Source: CAD feature listing. Evaluate the final solid. Frame: model axes, mm. Coordinates: 2 decimals unless noted, no trailing zeros. Loops run counter-clockwise (first coordinate to the right, second up) from the corner with the lowest first, then second, coordinate; pieces in that order, holes last. Notation, with made-up numbers: (25.25, 60.5) - (59.25, 60.5) arc R36 ccw to (59.25, 98.5) - close; hole circle Ø3 at (-34, 33.5). An arc over 180 degrees is marked (long way). Use one line per item in the form item = value. Start each with the question number.
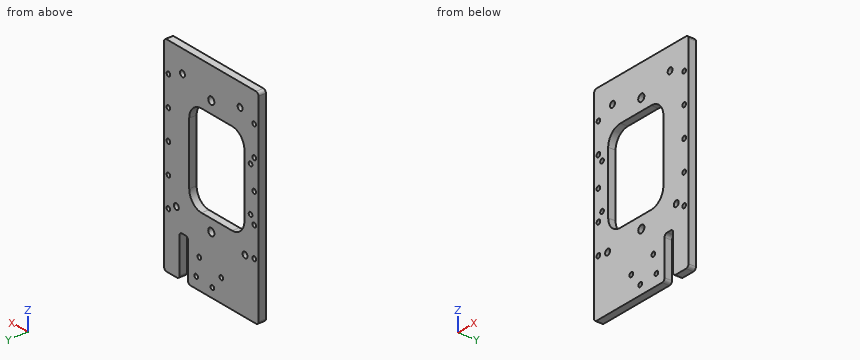
from build123d import *

# Parameters (mm, degrees)
SKETCH_1_W          = 77
SKETCH_1_H          = 138
SKETCH_1_R          = 2.5
SKETCH_1_W_2        = 45
SKETCH_1_H_2        = 62
EXTRUDE_1_DEPTH     = 5
SKETCH_7_W          = 7
SKETCH_7_H          = 28
CUT_EXTRUDE_1_DEPTH = 6
MM_CLEARANCE_0_D    = 4
FILLET_1_R          = 10
FILLET_2_R          = 2
MM_TRANSITIONAL_0_D = 3
MM_CLEARANCE_0_2_D  = 3


with BuildPart() as part:
    # 草图1 → 凸台-拉伸1 (new body)
    with BuildSketch(Plane(origin=(0, 0, 0), x_dir=(1, 0, 0), z_dir=(0, 1, 0))):
        with Locations((0, 9)):
            Rectangle(SKETCH_1_W, SKETCH_1_H)
        with Locations((0, 39)):
            Circle(SKETCH_1_R, mode=Mode.SUBTRACT)
        with Locations((0, -39)):
            Circle(SKETCH_1_R, mode=Mode.SUBTRACT)
        with Locations((-4.5, 0)):
            Rectangle(SKETCH_1_W_2, SKETCH_1_H_2, mode=Mode.SUBTRACT)
    extrude(amount=EXTRUDE_1_DEPTH)

    # 草图7 → 切除-拉伸1 (cut, through all)
    with BuildSketch(Plane(origin=(0, 5, 0), x_dir=(1, 0, 0), z_dir=(0, 1, 0))):
        with Locations((22.5, 64)):
            Rectangle(SKETCH_7_W, SKETCH_7_H)
    extrude(amount=-CUT_EXTRUDE_1_DEPTH, mode=Mode.SUBTRACT)

    # mm Clearance _0 (through all)
    with Locations(Plane(origin=(0, 0, 0), x_dir=(-1, 0, 0), z_dir=(0, -1, 0))):
        with Locations((-28.5, 36), (27.5, 41), (23.5, -45), (-23.5, -45)):
            Hole(MM_CLEARANCE_0_D / 2)

    # 圆角1
    fillet_1_edges = [part.edges().sort_by_distance(p)[0] for p in [
        (-27, 2.5, -31),
        (-27, 2.5, 31),
        (18, 2.5, 31),
        (18, 2.5, -31),
    ]]
    fillet(fillet_1_edges, radius=FILLET_1_R)

    # 圆角2
    fillet_2_edges = [part.edges().sort_by_distance(p)[0] for p in [
        (19, 2.5, -50),
        (19, 2.5, -78),
        (26, 2.5, -78),
        (26, 2.5, -50),
        (38.5, 2.5, 60),
        (-38.5, 2.5, 60),
        (-38.5, 2.5, -78),
        (38.5, 2.5, -78),
    ]]
    fillet(fillet_2_edges, radius=FILLET_2_R)

    # 大小mm Transitional 暗销孔0 (through all)
    with Locations(Plane(origin=(0, 5, 0), x_dir=(1, 0, 0), z_dir=(0, 1, 0))):
        with Locations((-31.999999999, 15), (-31.999999999, -15), (-8.142857142, 62.612808878), (-0.857142857, 71.612808878), (12.309431, 70.612808878), (9.80943136, 58.112808878)):
            Hole(MM_TRANSITIONAL_0_D / 2)

    # mm Clearance _0 2 (through all)
    with Locations(Plane(origin=(0, 5, 0), x_dir=(1, 0, 0), z_dir=(0, 1, 0))):
        with Locations((-35, 0), (-35, 20), (-35, 40), (-35, -40), (-35, -20), (35, 40), (35, 20), (35, 0), (35, -20), (35, -40)):
            Hole(MM_CLEARANCE_0_2_D / 2)


solid = part.part
(1) Contact query for a flat-ended pin moving along its axis: pin 1 (0.9 mm diameter, centred on x = 22, y = 1.5, fed in from -Z). Output: stop coordinate, or through.
(2) Cut plane C-C, the plane y = 2.7. State how many separate pieces and enclosed holes the cut face has, plus the area to 3 significant figures.
(3) Cut plane B-B, the plane x = -35. Output: boundary loops of the cut face in (y, z).
(4) Cut plane A-A, the plane z = 15. Output: boundary loops of the cut face in (x, y), plus the area to 3 significant figures.
(5) Material intervals for line 1 (Z direction, x = 35, y = 1.4); line 2 (Z direction, x = -6, y = 3.6); line 3 (X direction, y = 2.5, z = 45), sorted ascending.
Recorded:
q1.pin_1 = -50
q2.separate_pieces = 1
q2.enclosed_holes = 23
q2.area = 7,520 mm²
q3.outline = (0, -78) - (5, -78) - (5, -41.5) - (0, -41.5) - close; (0, -38.5) - (5, -38.5) - (5, -21.5) - (0, -21.5) - close; (0, -18.5) - (5, -18.5) - (5, -1.5) - (0, -1.5) - close; (0, 1.5) - (5, 1.5) - (5, 18.5) - (0, 18.5) - close; (0, 21.5) - (5, 21.5) - (5, 38.5) - (0, 38.5) - close; (0, 41.5) - (5, 41.5) - (5, 60) - (0, 60) - close
q4.outline = (-38.5, 0) - (-33.5, 0) - (-33.5, 5) - (-38.5, 5) - close; (-30.5, 0) - (-27, 0) - (-27, 5) - (-30.5, 5) - close; (18, 0) - (38.5, 0) - (38.5, 5) - (18, 5) - close
q4.area = 145 mm²
q5.line_1 = -78 to -41.5, -38.5 to -21.5, -18.5 to -1.5, 1.5 to 18.5, 21.5 to 38.5, 41.5 to 60
q5.line_2 = -78 to -31, 31 to 60
q5.line_3 = -38.5 to -25.5, -21.5 to 21.5, 25.5 to 38.5
